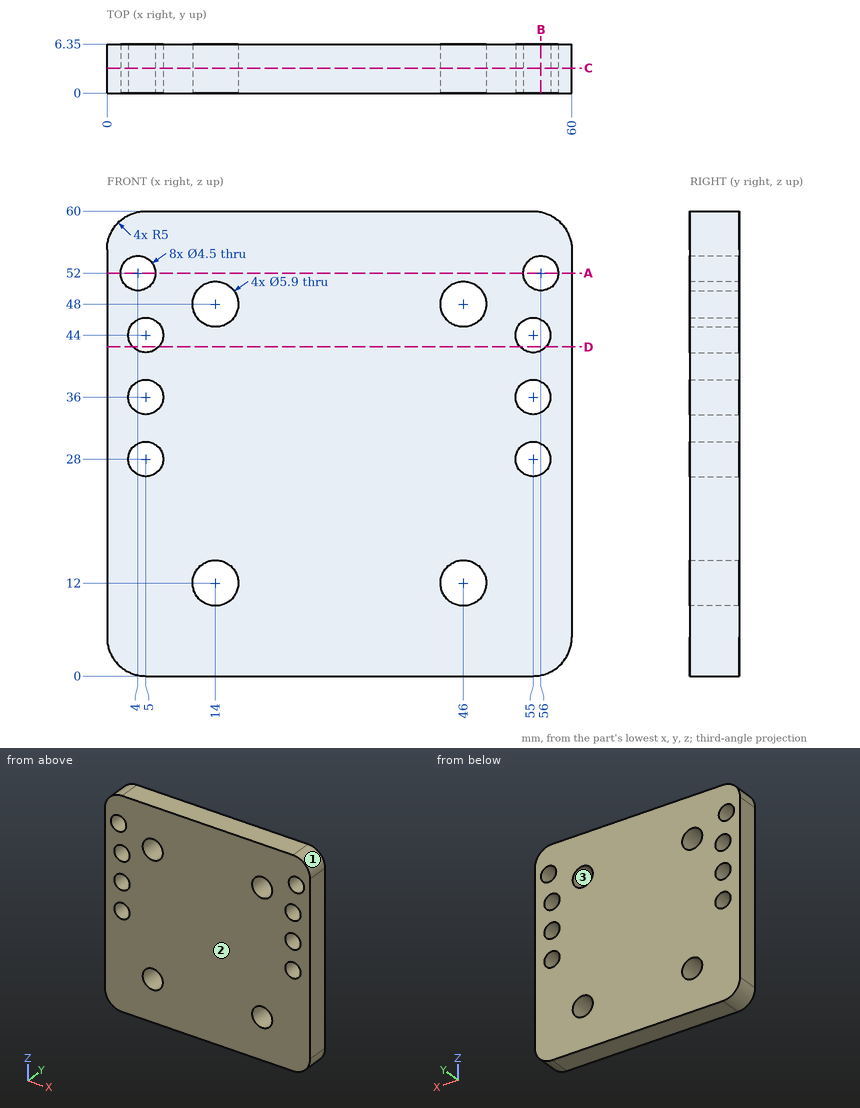
The figure shows three views and two pictorial views of one solid part (mm, origin at its lowest corner). Answer the questions. Round coordinates to 2 decimals unless told otherwise and drop trailing zeros. Order: outer loops, then holes, each group sorted by start corner. A loop starts at its lowest first (then second) coordinate and runs counter-clockwise, first axis right, second up. Notation, with made-up numbers: (46, -2) - (64, -2) arc R4 cw to (64, 4) - close; hole circle Ø10 at (33.5, 69.5). An arc over 180 degrees is marked (long way). Write item = value, one per line. Start each with the question number.
1) Section B-B, the plane x = 56 is taken. Write down the section's boundary in (y, z), plus the area to 3 significant figures.
2) Straight lines are drawn through the part: L1, parallel to X at y = 4.25, z = 52; L2, parallel to X at y = 4.5, z = 12; L3, parallel to Z at x = 7, y = 5.5. For each, find the intervals that lie inside material, in ascending order.
3) Section C-C, the plane y = 3.25 is taken. Count the separate pieces of the cut face and the enclosed holes in it, plus the area to 3 significant figures.
4) For a pull along X with two mould halves and no side action, classify the marked faces 1, 2 and 3 as released by +X, released by -X, zero draft, split by the parting line, or undercut.
5) Section A-A, the plane z = 52 is taken. Write down the section's boundary in (x, y), plus the area to 3 significant figures.
6) Section D-D, the plane z = 42.5 is taken. Write down the section's boundary in (x, y).
Results list:
q1.outline = (0, 0.1) - (6.35, 0.1) - (6.35, 25.98) - (0, 25.98) - close; (0, 30.02) - (6.35, 30.02) - (6.35, 33.98) - (0, 33.98) - close; (0, 38.02) - (6.35, 38.02) - (6.35, 41.98) - (0, 41.98) - close; (0, 46.02) - (6.35, 46.02) - (6.35, 49.75) - (0, 49.75) - close; (0, 54.25) - (6.35, 54.25) - (6.35, 59.9) - (0, 59.9) - close
q1.area = 274 mm^2
q2.L1 = 0 to 1.75, 6.25 to 53.75, 58.25 to 60
q2.L2 = 0 to 11.05, 16.95 to 43.05, 48.95 to 60
q2.L3 = 0 to 26.97, 29.03 to 34.97, 37.03 to 42.97, 45.03 to 60
q3.separate_pieces = 1
q3.enclosed_holes = 12
q3.area = 3,340 mm^2
q4.face_1 = released by +X
q4.face_2 = zero draft
q4.face_3 = undercut
q5.outline = (0, 0) - (1.75, 0) - (1.75, 6.35) - (0, 6.35) - close; (6.25, 0) - (53.75, 0) - (53.75, 6.35) - (6.25, 6.35) - close; (58.25, 0) - (60, 0) - (60, 6.35) - (58.25, 6.35) - close
q5.area = 324 mm^2
q6.outline = (0, 0) - (3.32, 0) - (3.32, 6.35) - (0, 6.35) - close; (6.68, 0) - (53.32, 0) - (53.32, 6.35) - (6.68, 6.35) - close; (56.68, 0) - (60, 0) - (60, 6.35) - (56.68, 6.35) - close
